Read the model definition and answer for the solid it produces. Units are mm, in the model's axes. A direction names the side the tool comes from. Coordinates: 2 decimals unless noted, no trailing zeros. Order: outer loops, then holes, each group sorted by start corner. A loop starts at its lowest first (then second) coordinate and runs counter-clockwise, first axis right, second up. Notation, with made-up numbers: M 32.25,59.5 L 43.25,59.5 A20 ccw 43.25,98.5 Z; hole C 22.5,6.5 d2. An arc over 180 degrees is marked long. One line per question, with ' | ' between items. Start each with the question number.
1) Find section B-B, the plane x = 0. Write down the section's boundary in (y, z), plus the area to 3 significant figures.
2) Find section A-A, the plane z = 39.5. Write down the section's boundary in (x, y).
3) Find section D-D, the plane x = -50. Write down the section's boundary in (y, z), plus the area to 3 significant figures.
4) Given P1, Ø1.5, axis at x = 29.5, y = 73, coming from the -Z side; P2, Ø12, axis at y = 91, z = 10, coming from the +X side; P3, Ø20, axis at x = 72, z = 12.5, coming from the +Y side, each flat-ended and moving along its own axis, determine where each tip first touches the part or whether it passes through.
5) The mould has two halves that part along X. Classify faces 6 (the face through (-97.32, 7.4, -19.63)), 7 (the face through (60, 7, 30)), 8 (the face through (99.54, 7.4, -26.39)): +X half, -X half, draft (parallel to the pull), parting line (faces both ways), or undercut.
6) Consider probe 1 along Y at (x, z) = (0, 10); probe 2 along X at (y, z) = (10, 18); probe 3 along X at (y, z) = (6, 18). Determine where each line is inside the solid, lowest interval first.
7) Find section C-C, the plane y = 100. Write down the section's boundary in (x, z), plus the area to 3 significant figures.
8) A tool of negligible diameter and unlimited length cuts with its end or side. For faces 1 (the face through (66, 15, -18)), 2 (the face through (-67, 15, 17)), 3 (the face through (66, 15, 17)), 4 (the face through (-44, 44, 5)), 5 (the face through (0, 63, 45)), from which of +Z, -Z, +X, -X, +Y, -Y can it reach the whole face along a straight path? Write none if from no direction.
from build123d import *
from build123d.topology import SkipClean

# Parameters (mm, degrees)
SKETCH1_R           = 15
BOSS_EXTRUDE1_DEPTH = 45
SKETCH4_R           = 7.5
BOSS_EXTRUDE2_DEPTH = 15
CUT_EXTRUDE1_DEPTH  = 179.469413089
BOSS_EXTRUDE3_DEPTH = 5


with BuildPart() as part:
    # Sketch1 → Boss-Extrude1 (new, symmetric)
    with BuildSketch(Plane.XY):
        with BuildLine():
            ThreePointArc((-5, 33.400370285), (-25.587569792, 22.042255042), (-33.772544103, 0))
            Line((-33.772544103, 0), (-18.781429719, 0))
            ThreePointArc((-18.781429719, 0), (0, 18.781429719), (18.781429719, 0))
            Line((18.781429719, 0), (33.772544103, 0))
            ThreePointArc((33.772544103, 0), (25.587569792, 22.042255042), (5, 33.400370285))
            Line((5, 33.400370285), (5, 75.505102572))
            ThreePointArc((5, 75.505102572), (0, 125), (-5, 75.505102572))
            Line((-5, 75.505102572), (-5, 33.400370285))
        make_face()
        with Locations(Location((0, 100, 0), (0, 0, 180))):
            Circle(SKETCH1_R, mode=Mode.SUBTRACT)
    extrude(amount=BOSS_EXTRUDE1_DEPTH, both=True)

    # Sketch4 → Boss-Extrude2 (add)
    with BuildSketch(Plane(origin=(0, 0, 0), x_dir=(1, 0, 0), z_dir=(0, 1, 0))):
        with BuildLine():
            Line((-90.962767097, -30), (90.962767097, -30))
            ThreePointArc((90.962767097, -30), (99.448048472, -26.485281374), (102.962767097, -18))
            Line((102.962767097, -18), (102.962767097, 18))
            ThreePointArc((102.962767097, 18), (99.448048472, 26.485281374), (90.962767097, 30))
            Line((90.962767097, 30), (-90.962767097, 30))
            ThreePointArc((-90.962767097, 30), (-99.448048472, 26.485281374), (-102.962767097, 18))
            Line((-102.962767097, 18), (-102.962767097, -18))
            ThreePointArc((-102.962767097, -18), (-99.448048472, -26.485281374), (-90.962767097, -30))
        make_face()
        with Locations(Location((-90, 18, 0), (0, 0, 270))):
            Circle(SKETCH4_R, mode=Mode.SUBTRACT)
        with Locations(Location((90, 18, 0), (0, 0, 90))):
            Circle(SKETCH4_R, mode=Mode.SUBTRACT)
        with Locations(Location((90, -18, 0), (0, 0, 270))):
            Circle(SKETCH4_R, mode=Mode.SUBTRACT)
        with Locations(Location((-90, -18, 0), (0, 0, 90))):
            Circle(SKETCH4_R, mode=Mode.SUBTRACT)
    extrude(amount=BOSS_EXTRUDE2_DEPTH)

    # Sketch5 → Cut-Extrude1 (cut, through all)
    with SkipClean():  # the faces are left unmerged after this step: merging them gives an invalid solid
        with BuildSketch(Plane.XY.offset(30)):
            with BuildLine():
                Line((-18.781429719, 0), (18.781429719, 0))
                ThreePointArc((18.781429719, 0), (16.807967644, 8.380592221), (11.302305177, 15))
                Line((11.302305177, 15), (-11.302305177, 15))
                ThreePointArc((-11.302305177, 15), (-16.807967644, 8.380592221), (-18.781429719, 0))
            make_face()
        extrude(amount=-CUT_EXTRUDE1_DEPTH, mode=Mode.SUBTRACT)
    add(part.part.scale(1), mode=Mode.REPLACE)  # the faces are merged on a copy

    # Sketch6 → Boss-Extrude3 (add, symmetric)
    with SkipClean():  # the faces are left unmerged after this step: merging them gives an invalid solid
        with BuildSketch(Plane.XY):
            with BuildLine():
                Line((102.962767097, 15), (19.244209313, 115.95808284))
                ThreePointArc((19.244209313, 115.95808284), (23.580846559, 91.696767162), (5, 75.505102572))
                Line((5, 75.505102572), (5, 33.400370285))
                ThreePointArc((5, 33.400370285), (19.885576867, 27.297409545), (30.258630755, 15))
                Line((30.258630755, 15), (90.962767097, 15))
                Line((90.962767097, 15), (102.962767097, 15))
            make_face()
            with BuildLine():
                ThreePointArc((-5, 75.505102572), (-23.580846559, 91.696767162), (-19.244209313, 115.95808284))
                Line((-19.244209313, 115.95808284), (-102.962767097, 15))
                Line((-102.962767097, 15), (-90.962767097, 15))
                Line((-90.962767097, 15), (-30.258630755, 15))
                ThreePointArc((-30.258630755, 15), (-19.885576867, 27.297409545), (-5, 33.400370285))
                Line((-5, 33.400370285), (-5, 75.505102572))
            make_face()
        extrude(amount=BOSS_EXTRUDE3_DEPTH, both=True)


solid = part.part
Report:
1) outline: M 18.78,-45 L 85,-45 L 85,45 L 18.78,45 Z; M 115,-45 L 125,-45 L 125,45 L 115,45 Z | area: 6,860 mm^2
2) outline: M -33.77,0 L -18.78,0 A18.78 cw 18.78,0 L 33.77,0 A33.77 ccw 5,33.4 L 5,75.51 A25 ccw long -5,75.51 L -5,33.4 A33.77 ccw Z; hole C 0,100 d30
3) outline: M 0,-30 L 15,-30 L 15,-5 L 78.87,-5 L 78.87,5 L 15,5 L 15,30 L 0,30 Z | area: 1,540 mm^2
4) P1: stops at z = -5 | P2: stops at x = 42.69 | P3: stops at y = 60.32
5) face 6: undercut | face 7: draft | face 8: +X half
6) probe 1: y = 18.78 to 85, 115 to 125 | probe 2: x = -102.96 to -97.5, -82.5 to -15.9, 15.9 to 82.5, 97.5 to 102.96 | probe 3: x = -102.96 to -97.5, -82.5 to -17.8, 17.8 to 82.5, 97.5 to 102.96
7) outline: M -32.48,-5 L -25,-5 L -25,-45 L -15,-45 L -15,45 L -25,45 L -25,5 L -32.48,5 Z; M 15,-45 L 25,-45 L 25,-5 L 32.48,-5 L 32.48,5 L 25,5 L 25,45 L 15,45 Z | area: 1,950 mm^2
8) face 1: -Z, +X, +Y | face 2: +Z, -X, +Y | face 3: +Z, +X, +Y | face 4: +Z, -X | face 5: +Z, +X, -X, +Y, -Y
